Read the model definition and answer for the solid it produces. Units are mm, in the model's axes. A direction names the side the tool comes from. Give positions to 0.01 mm unless a question says otherwise; leave off trailing zeros. Loops run counter-clockwise (first coordinate to the right, second up) from the corner with the lowest first, then second, coordinate; pieces in that order, holes last. Notation, with made-up numbers: (14.25, 35) -> (39.25, 35) arc R29 ccw to (39.25, 57) -> close; hole circle Ø3 at (60, 17.25). An arc over 180 degrees is marked (long way). Return JSON: item names as keys, results as strings. Group by question number.
from build123d import *

# Parameters (mm, degrees)
SKETCH1_W                                            = 300
SKETCH1_H                                            = 210
BOSS_EXTRUDE1_DEPTH                                  = 10
SKETCH2_W                                            = 280
SKETCH2_H                                            = 190
BOSS_EXTRUDE2_DEPTH                                  = 9.28
F_1_4_20_CLEARANCE_HOLES_REACH                       = 21.28
SKETCH3_R                                            = 3.57
SKETCH4_R                                            = 7.5
CUT_EXTRUDE2_DEPTH                                   = 10
SKETCH11_W                                           = 54
SKETCH11_H                                           = 51
TEC_DEPTH                                            = 1
FILLET1_R                                            = 2
F_4_40_TAPPED_HOLE1_D                                = 2.2606
F_4_40_TAPPED_HOLE1_DEPTH                            = 13
F_4_40_TAPPED_HOLE1_TIP                              = 0.679152758
F_4_40_TAPPED_HOLE2_D                                = 2.2606
F_4_40_TAPPED_HOLE2_DEPTH                            = 13
F_4_40_TAPPED_HOLE2_TIP                              = 0.679152758
F_4_40_TAPPED_HOLE3_D                                = 2.2606
F_4_40_TAPPED_HOLE3_DEPTH                            = 13
F_4_40_TAPPED_HOLE3_TIP                              = 0.679152758
F_4_40_TAPPED_HOLE4_D                                = 2.2606
F_4_40_TAPPED_HOLE4_DEPTH                            = 13
F_4_40_TAPPED_HOLE4_TIP                              = 0.679152758
CBORE_FOR_1_4_BINDING_HEAD_MACHINE_SCREW_D           = 6.7564
CBORE_FOR_1_4_BINDING_HEAD_MACHINE_SCREW_CBORE_D     = 14.2875
CBORE_FOR_1_4_BINDING_HEAD_MACHINE_SCREW_CBORE_DEPTH = 4.191


with BuildPart() as part:
    # Sketch1 → Boss-Extrude1 (new body)
    with BuildSketch(Plane(origin=(0, 0, 0), x_dir=(1, 0, 0), z_dir=(0, 1, 0))):
        with Locations((-22.864321608, -2.487437186)):
            Rectangle(SKETCH1_W, SKETCH1_H)
    extrude(amount=BOSS_EXTRUDE1_DEPTH)

    # Sketch2 → Boss-Extrude2 (add)
    with BuildSketch(Plane(origin=(0, 10, 0), x_dir=(1, 0, 0), z_dir=(0, 1, 0))):
        with Locations((-22.864321608, -2.487437186)):
            Rectangle(SKETCH2_W, SKETCH2_H)
    extrude(amount=BOSS_EXTRUDE2_DEPTH)

    # Sketch3 → 1/4-20 clearance holes (cut, up to next)
    with BuildSketch(Plane(origin=(0, 19.28, 0), x_dir=(1, 0, 0), z_dir=(0, 1, 0)), mode=Mode.PRIVATE) as f_1_4_20_clearance_holes_sk1:
        with Locations((-122.864321608, 65.012562814)):
            Circle(SKETCH3_R)
    f_1_4_20_clearance_holes_tool1 = extrude(f_1_4_20_clearance_holes_sk1.sketch, amount=-F_1_4_20_CLEARANCE_HOLES_REACH, mode=Mode.PRIVATE) & part.part
    add(f_1_4_20_clearance_holes_tool1.solids().sort_by_distance((-122.864322, 19.28, -65.012563))[0], mode=Mode.SUBTRACT)
    # Sketch3 → 1/4-20 clearance holes (cut, up to next)
    with BuildSketch(Plane(origin=(0, 19.28, 0), x_dir=(1, 0, 0), z_dir=(0, 1, 0)), mode=Mode.PRIVATE) as f_1_4_20_clearance_holes_sk2:
        with Locations((-39.114321608, 65.012562814)):
            Circle(SKETCH3_R)
    f_1_4_20_clearance_holes_tool2 = extrude(f_1_4_20_clearance_holes_sk2.sketch, amount=-F_1_4_20_CLEARANCE_HOLES_REACH, mode=Mode.PRIVATE) & part.part
    add(f_1_4_20_clearance_holes_tool2.solids().sort_by_distance((-39.114322, 19.28, -65.012563))[0], mode=Mode.SUBTRACT)
    # Sketch3 → 1/4-20 clearance holes (cut, up to next)
    with BuildSketch(Plane(origin=(0, 19.28, 0), x_dir=(1, 0, 0), z_dir=(0, 1, 0)), mode=Mode.PRIVATE) as f_1_4_20_clearance_holes_sk3:
        with Locations((44.635678392, 65.012562814)):
            Circle(SKETCH3_R)
    f_1_4_20_clearance_holes_tool3 = extrude(f_1_4_20_clearance_holes_sk3.sketch, amount=-F_1_4_20_CLEARANCE_HOLES_REACH, mode=Mode.PRIVATE) & part.part
    add(f_1_4_20_clearance_holes_tool3.solids().sort_by_distance((44.635678, 19.28, -65.012563))[0], mode=Mode.SUBTRACT)
    # Sketch3 → 1/4-20 clearance holes (cut, up to next)
    with BuildSketch(Plane(origin=(0, 19.28, 0), x_dir=(1, 0, 0), z_dir=(0, 1, 0)), mode=Mode.PRIVATE) as f_1_4_20_clearance_holes_sk4:
        with Locations((44.635678392, -69.987437186)):
            Circle(SKETCH3_R)
    f_1_4_20_clearance_holes_tool4 = extrude(f_1_4_20_clearance_holes_sk4.sketch, amount=-F_1_4_20_CLEARANCE_HOLES_REACH, mode=Mode.PRIVATE) & part.part
    add(f_1_4_20_clearance_holes_tool4.solids().sort_by_distance((44.635678, 19.28, 69.987437))[0], mode=Mode.SUBTRACT)
    # Sketch3 → 1/4-20 clearance holes (cut, up to next)
    with BuildSketch(Plane(origin=(0, 19.28, 0), x_dir=(1, 0, 0), z_dir=(0, 1, 0)), mode=Mode.PRIVATE) as f_1_4_20_clearance_holes_sk5:
        with Locations((-39.114321608, -69.987437186)):
            Circle(SKETCH3_R)
    f_1_4_20_clearance_holes_tool5 = extrude(f_1_4_20_clearance_holes_sk5.sketch, amount=-F_1_4_20_CLEARANCE_HOLES_REACH, mode=Mode.PRIVATE) & part.part
    add(f_1_4_20_clearance_holes_tool5.solids().sort_by_distance((-39.114322, 19.28, 69.987437))[0], mode=Mode.SUBTRACT)
    # Sketch3 → 1/4-20 clearance holes (cut, up to next)
    with BuildSketch(Plane(origin=(0, 19.28, 0), x_dir=(1, 0, 0), z_dir=(0, 1, 0)), mode=Mode.PRIVATE) as f_1_4_20_clearance_holes_sk6:
        with Locations((-122.864321608, -69.987437186)):
            Circle(SKETCH3_R)
    f_1_4_20_clearance_holes_tool6 = extrude(f_1_4_20_clearance_holes_sk6.sketch, amount=-F_1_4_20_CLEARANCE_HOLES_REACH, mode=Mode.PRIVATE) & part.part
    add(f_1_4_20_clearance_holes_tool6.solids().sort_by_distance((-122.864322, 19.28, 69.987437))[0], mode=Mode.SUBTRACT)

    # Sketch4 → Cut-Extrude2 (cut)
    with BuildSketch(Plane.XZ):
        with Locations((-122.864321608, 69.987437186)):
            Circle(SKETCH4_R)
        with Locations((-39.114321608, 69.987437186)):
            Circle(SKETCH4_R)
        with Locations((44.635678392, 69.987437186)):
            Circle(SKETCH4_R)
        with Locations((44.635678392, -65.012562814)):
            Circle(SKETCH4_R)
        with Locations((-39.114321608, -65.012562814)):
            Circle(SKETCH4_R)
        with Locations((-122.864321608, -65.012562814)):
            Circle(SKETCH4_R)
    extrude(amount=-CUT_EXTRUDE2_DEPTH, mode=Mode.SUBTRACT)

    # Sketch11 → TEC (cut)
    with BuildSketch(Plane(origin=(0, 19.28, 0), x_dir=(1, 0, 0), z_dir=(0, 1, 0))):
        with Locations((-66.114321608, 24.512562814)):
            Rectangle(SKETCH11_W, SKETCH11_H)
        with Locations((-80.864321608, -44.487437186)):
            Rectangle(SKETCH11_W, SKETCH11_H)
        with Locations((2.635678392, -44.487437186)):
            Rectangle(SKETCH11_W, SKETCH11_H)
    extrude(amount=-TEC_DEPTH, mode=Mode.SUBTRACT)

    # Fillet1
    fillet1_edges = [part.edges().sort_by_distance(p)[0] for p in [
        (29.635678392, 18.78, 69.987437186),
        (-24.364321608, 18.78, 69.987437186),
        (-24.364321608, 18.78, 18.987437186),
        (29.635678392, 18.78, 18.987437186),
        (-39.114321608, 18.78, -50.012562814),
        (-39.114321608, 18.78, 0.987437186),
        (-93.114321608, 18.78, 0.987437186),
        (-93.114321608, 18.78, -50.012562814),
        (-53.864321608, 18.78, 69.987437186),
        (-107.864321608, 18.78, 69.987437186),
        (-107.864321608, 18.78, 18.987437186),
        (-53.864321608, 18.78, 18.987437186),
    ]]
    fillet(fillet1_edges, radius=FILLET1_R)

    # #4-40 Tapped Hole1
    with Locations(Plane.ZY.offset(162.864321608)):
        with Locations((-62.512562814, 14.64), (2.487437186, 14.64), (67.487437186, 14.64)):
            Hole(F_4_40_TAPPED_HOLE1_D / 2, depth=F_4_40_TAPPED_HOLE1_DEPTH)
            with Locations((0, 0, -(F_4_40_TAPPED_HOLE1_DEPTH + F_4_40_TAPPED_HOLE1_TIP / 2))):  # 118° drill point
                Cone(0, F_4_40_TAPPED_HOLE1_D / 2, F_4_40_TAPPED_HOLE1_TIP, mode=Mode.SUBTRACT)

    # #4-40 Tapped Hole2
    with Locations(Plane.XY.offset(97.487437186)):
        with Locations((-147.864321608, 14.64), (-22.864321608, 14.64), (102.135678392, 14.64)):
            Hole(F_4_40_TAPPED_HOLE2_D / 2, depth=F_4_40_TAPPED_HOLE2_DEPTH)
            with Locations((0, 0, -(F_4_40_TAPPED_HOLE2_DEPTH + F_4_40_TAPPED_HOLE2_TIP / 2))):  # 118° drill point
                Cone(0, F_4_40_TAPPED_HOLE2_D / 2, F_4_40_TAPPED_HOLE2_TIP, mode=Mode.SUBTRACT)

    # #4-40 Tapped Hole3
    with Locations(Plane(origin=(117.135678392, 0, 0), x_dir=(0, 0, -1), z_dir=(1, 0, 0))):
        with Locations((-67.487437186, 14.64), (-2.487437186, 14.64), (62.512562814, 14.64)):
            Hole(F_4_40_TAPPED_HOLE3_D / 2, depth=F_4_40_TAPPED_HOLE3_DEPTH)
            with Locations((0, 0, -(F_4_40_TAPPED_HOLE3_DEPTH + F_4_40_TAPPED_HOLE3_TIP / 2))):  # 118° drill point
                Cone(0, F_4_40_TAPPED_HOLE3_D / 2, F_4_40_TAPPED_HOLE3_TIP, mode=Mode.SUBTRACT)

    # #4-40 Tapped Hole4
    with Locations(Plane(origin=(0, 0, -92.512562814), x_dir=(-1, 0, 0), z_dir=(0, 0, -1))):
        with Locations((-102.135678392, 14.64), (22.864321608, 14.64), (147.864321608, 14.64)):
            Hole(F_4_40_TAPPED_HOLE4_D / 2, depth=F_4_40_TAPPED_HOLE4_DEPTH)
            with Locations((0, 0, -(F_4_40_TAPPED_HOLE4_DEPTH + F_4_40_TAPPED_HOLE4_TIP / 2))):  # 118° drill point
                Cone(0, F_4_40_TAPPED_HOLE4_D / 2, F_4_40_TAPPED_HOLE4_TIP, mode=Mode.SUBTRACT)

    # CBORE for 1/4 Binding Head Machine Screw1 (through all)
    with Locations(Plane(origin=(0, 19.28, 0), x_dir=(1, 0, 0), z_dir=(0, 1, 0))):
        with Locations((80.735678392, 61.012562814), (80.735678392, -65.987437186), (-147.864321608, 35.612562814), (-147.864321608, -40.587437186)):
            CounterBoreHole(CBORE_FOR_1_4_BINDING_HEAD_MACHINE_SCREW_D / 2, CBORE_FOR_1_4_BINDING_HEAD_MACHINE_SCREW_CBORE_D / 2, CBORE_FOR_1_4_BINDING_HEAD_MACHINE_SCREW_CBORE_DEPTH)


solid = part.part
1. Determine the mould class of faces 1 (the flat face through (-25, 5, -102.513)), 2 (the flat face through (-35, 10, 103)), 3 (the cylindrical face through (84.11, 7.44, -61.16)) for opening direction Z: pulls with the +Z half, pulls with the -Z half, needs draft (parallel to the pull), parting line crosses it, or undercut.
2. Which of the six approach directions +Z, -Z, +X, -X, +Y, -Y give full straight-line access (tool end or side, diameter ignored) to faces 4 (the flat face through (-162.864, 15, 4)), 5 (the flat face through (-81, 18.28, 44)), 6 (the flat face through (-119.6, 10, 71.8)), 7 (the cylindrical face through (-151.087, 7.439, 39.573))?
3. Straight lines are drawn through the part: line 1 (Z direction, x = -153, y = 14.64); line 2 (X direction, y = 14.64, z = -83); line 3 (X direction, y = 17.25, z = -62). For each, find the intervals that lie inside material, in ascending order. Write a range as from..to.
4. Section A-A on x = 57.5 is taken. Determine the outline of the cut face in (y, z).
5. Section C-C on x = -63 is taken. Determine the outline of the cut face in (y, z), then the cut area to 3 significant figures.
6. Section B-B on x = -100.5 is taken. Determine the outline of the cut face in (y, z).
7. Flat-ended cylindrical pins translate along their axes: pin 1 Ø1.5 at (y, z) = (11.5, 70.5) entering from -X; pin 2 Ø9.5 at (x, z) = (44.64, -65.01) entering from -Y; pin 3 Ø2 at (x, y) = (-147.86, 14.64) entering from +Z; pin 4 Ø5.5 at (x, z) = (-122.86, -65.01) entering from +Y. Find the tip coordinate at first contact, or state that the pin passes through.
Completed:
{
 "1": {"face 1": "pulls with the -Z half", "face 2": "needs draft", "face 3": "undercut"},
 "2": {"face 4": "+Z, -Z, -X, +Y", "face 5": "+Y", "face 6": "-Y", "face 7": "+Y, -Y"},
 "3": {"line 1": "z = -92.51..-63.64, -61.38..1.36, 3.62..66.36, 68.62..97.49", "line 2": "x = -162.86..-148.99, -146.73..-23.99, -21.73..101.01, 103.27..117.14", "line 3": "x = -162.86..-124.78, -120.95..-41.03, -37.2..42.72, 46.55..73.66, 87.81..117.14"},
 "4": {"outline": "(0, -102.51) -> (10, -102.51) -> (10, -92.51) -> (19.28, -92.51) -> (19.28, 97.49) -> (10, 97.49) -> (10, 107.49) -> (0, 107.49) -> close"},
 "5": {"outline": "(0, -102.51) -> (10, -102.51) -> (10, -92.51) -> (19.28, -92.51) -> (19.28, -50.01) -> (18.28, -50.01) -> (18.28, 0.99) -> (19.28, 0.99) -> (19.28, 18.99) -> (18.28, 18.99) -> (18.28, 69.99) -> (19.28, 69.99) -> (19.28, 97.49) -> (10, 97.49) -> (10, 107.49) -> (0, 107.49) -> close", "area": "3,760 mm²"},
 "6": {"outline": "(0, -102.51) -> (10, -102.51) -> (10, -92.51) -> (19.28, -92.51) -> (19.28, 18.99) -> (18.28, 18.99) -> (18.28, 69.99) -> (19.28, 69.99) -> (19.28, 97.49) -> (10, 97.49) -> (10, 107.49) -> (0, 107.49) -> close"},
 "7": {"pin 1": "stops at x = -162.86", "pin 2": "stops at y = 10", "pin 3": "stops at z = 84.41", "pin 4": "passes through"}
}
